Autodesk Inventor part; units mm, degrees
ref_plane "YZ Plane" through (0, 0, 0) normal (1, 0, 0) x (0, 1, 0)
ref_plane "XZ Plane" through (0, 0, 0) normal (0, 1, 0) x (-1, 0, 0)
ref_plane "XY Plane" through (0, 0, 0) normal (0, 0, 1) x (1, 0, 0)
sketch "Sketch1" plane through (0, 0, 0) normal (0, 1, 0) x (-1, 0, 0)
  circle A0 centre (0, 0) radius 3
  dimension "d0" = 6
extrude "Extrusion1" add sketch "Sketch1" along normal blind 5.5
sketch "Sketch2" plane through (0, 5.5, 0) normal (0, 1, 0) x (1, 0, 0)
  circle A0 centre (0, 0) radius 2
  dimension "d3" = 4
extrude "Extrusion2" add sketch "Sketch2" along normal blind 1.5
sketch "Sketch3" plane through (0, 7, 0) normal (0, 1, 0) x (1, 0, 0)
  circle A0 centre (0, 0) radius 4
  dimension "d6" = 8
extrude "Extrusion3" add sketch "Sketch3" along normal blind 11
sketch "Sketch4" plane through (0, 18, 0) normal (0, 1, 0) x (1, 0, 0)
  circle A0 centre (0, 0) radius 3
  dimension "d9" = 6
extrude "Extrusion4" add sketch "Sketch4" along normal blind 25
sketch "Sketch5" plane through (0, 43, 0) normal (0, 1, 0) x (1, 0, 0)
  circle A0 centre (0, 0) radius 3
  circle A1 centre (0, 0) radius 1.5
  dimension "d12" = 3
extrude "Extrusion5" add sketch "Sketch5" along normal blind 6 contours A1
thread "Thread1"
properties part number "reverse gear lever ring stud"
Geometry check sheet. Reference: the model listing, model coordinates, mm. A direction names the side the tool comes from. Give positions to 0.01 mm unless a question says otherwise; leave off trailing zeros. Loops run counter-clockwise (first coordinate to the right, second up) from the corner with the lowest first, then second, coordinate; pieces in that order, holes last. Notation, with made-up numbers: (-23.75, -13.75) -> (35.25, -13.75) arc R33 cw to (35.25, 15.25) -> close; hole circle Ø1 at (79.5, 81). An arc over 180 degrees is marked (long way). Answer in a Markdown table with one row per item. Add a question column.
1) Set-up check for faces 1 (the face through (-2, 7, 1)), 2 (the face through (-1.5, 45.96, 0.07)), 3 (the face through (3, 3, 0)): record each of +Z, -Z, +X, -X, +Y, -Y from which the full face is reachable in a straight line by a thin tool's end or side.
2) Material ranges on probe 1 along Y at (x, z) = (-2.25, -0.5); probe 2 along Y at (x, z) = (2.75, 2.5); probe 3 along X at (y, z) = (34.5, 0), recorded low to high. Write a range as from..to.
3) Gauge pin test, flat ends, axial feed: P1, Ø1.5, axis at x = 2.5, y = 12, coming from the +Z side; P2, Ø4, axis at x = 1, y = 27, coming from the -Z side; P3, Ø1.5, axis at y = 34, z = 1, coming from the +X side. Record the tip position at first contact, or that the pin passes through.
4) Cross-section at A-A on z = 0. Record the boundary of the cut face in (x, y), and give its area (3 significant figures).
5) Cross-section at C-C on y = 8. Record the boundary of the cut face in (x, z), and give its area (3 significant figures).
6) Cross-section at B-B on x = 1. Record the boundary of the cut face in (y, z).
Outcome:
| question | item | result |
|---|---|---|
| 1 | face 1 | none |
| 1 | face 2 | +Y |
| 1 | face 3 | -Y |
| 2 | probe 1 | y = 0..5.5, 7..43 |
| 2 | probe 2 | y = 7..18 |
| 2 | probe 3 | x = -3..3 |
| 3 | P1 | stops at z = 3.6 |
| 3 | P2 | stops at z = -3 |
| 3 | P3 | stops at x = 2.99 |
| 4 | outline | (-4, 7) -> (-2, 7) -> (-2, 5.5) -> (-3, 5.5) -> (-3, 0) -> (3, 0) -> (3, 5.5) -> (2, 5.5) -> (2, 7) -> (4, 7) -> (4, 18) -> (3, 18) -> (3, 43) -> (1.5, 43) -> (1.5, 49) -> (-1.5, 49) -> (-1.5, 43) -> (-3, 43) -> (-3, 18) -> (-4, 18) -> close |
| 4 | area | 295 mm^2 |
| 5 | outline | circle Ø8 at (0, 0) |
| 5 | area | 50.3 mm^2 |
| 6 | outline | (0, -2.83) -> (5.5, -2.83) -> (5.5, -1.73) -> (7, -1.73) -> (7, -3.87) -> (18, -3.87) -> (18, -2.83) -> (43, -2.83) -> (43, -1.12) -> (49, -1.12) -> (49, 1.12) -> (43, 1.12) -> (43, 2.83) -> (18, 2.83) -> (18, 3.87) -> (7, 3.87) -> (7, 1.73) -> (5.5, 1.73) -> (5.5, 2.83) -> (0, 2.83) -> close |
